Part model, mm, in its own coordinate system. A direction names the side the tool comes from. Coordinates: 2 decimals unless noted, no trailing zeros. Order: outer loops, then holes, each group sorted by start corner. A loop starts at its lowest first (then second) coordinate and runs counter-clockwise, first axis right, second up. Notation, with made-up numbers: (-6, 10.5) - (2, 10.5) arc R20 cw to (2, 42.5) - close; hole circle Ø9 at (-40, 30). An arc over 180 degrees is marked (long way). Use a Markdown table: item, result. Add a question column.
1) Saw through at B-B on x = 3. List the corners of the cut face in (y, z).
2) Drop flat-ended pins along their axis: P1, Ø6, axis at x = -5, y = 3, coming from the +Z side; P2, Ø2, axis at x = -3, y = -4, coming from the -Z side. Give the stop position or say it passes through.
3) Wall check: L1, parallel to Y at x = 1.5, z = 1.8; L2, parallel to Y at x = 1.75, z = 0.5; L3, parallel to X at y = 4.5, z = 0.7. Give the ranges that are in metal, low to high. Write a range as [from, to].
4) Tool access for faces 1 (the face through (1.39, 1.52, 2)), 2 (the face through (3.138, -3.702, 1.268)), 3 (the face through (-3.88, -7.31, 2)), 4 (the face through (-4.53, -7.12, 1.27)): list every direction of +Z, -Z, +X, -X, +Y, -Y with a clear straight run to the whole face (end or side of a thin tool).
5) Saw through at D-D on z = 2.15. List the corners of the cut face in (x, y), then the cut area to 3 significant figures.
6) Saw through at A-A on z = 0.3. List the corners of the cut face in (x, y), then the cut area to 3 significant figures.
7) Saw through at C-C on y = -6. List the corners of the cut face in (x, z), then the cut area to 3 significant figures.
```python
from build123d import *

# Parameters (mm, degrees)
F1_DEPTH = 2.54
F2_SIZE  = 1.0922
F3_SIZE  = 1.0922


with BuildPart() as f1:
    # F0 (on Top) → F1 (new body)
    with BuildSketch(Plane.XY):
        Polygon((3.7357374094, 2.0727487281), (1.6156566562, 6.3129104674), (-0.688809203, 5.7773781009), (0, 3.146545263), (-3.5388784017, 1.3378473232), (-1.3465175871, -4.636336118), (-7.8139826655, -9.6787661314), (-5.0735310651, -18.2837825269), (5.5594188161, -7.8152595088), (0.6475421183, 0.5286511673), align=None)
    extrude(amount=F1_DEPTH)

    # F2
    f2_edges = [f1.edges().sort_by_distance(p)[0] for p in [
        (3.10348, -3.643304, 2.54),
        (2.19164, 1.3007, 2.54),
        (2.675697, 4.19283, 2.54),
        (0.463424, 6.045144, 2.54),
        (-0.344405, 4.461962, 2.54),
        (-1.769439, 2.242196, 2.54),
        (-2.442698, -1.649244, 2.54),
        (-4.58025, -7.157551, 2.54),
        (-6.443757, -13.981274, 2.54),
        (0.242944, -13.049521, 2.54),
    ]]
    chamfer(f2_edges, length=F2_SIZE)

    # F3
    f3_edges = [f1.edges().sort_by_distance(p)[0] for p in [
        (3.10348, -3.643304, 0),
        (2.19164, 1.3007, 0),
        (2.675697, 4.19283, 0),
        (0.463424, 6.045144, 0),
        (-0.344405, 4.461962, 0),
        (-1.769439, 2.242196, 0),
        (-2.442698, -1.649244, 0),
        (-4.58025, -7.157551, 0),
        (-6.443757, -13.981274, 0),
        (0.242944, -13.049521, 0),
    ]]
    chamfer(f3_edges, length=F3_SIZE)


solid = f1.part
```
Results are:
| question | item | result |
|---|---|---|
| 1 | outline | (-10.34, 1.09) - (-8.8, 0) - (-5.62, 0) - (-3.47, 1.09) - (-3.47, 1.45) - (-5.62, 2.54) - (-8.8, 2.54) - (-10.34, 1.45) - close; (1.7, 1.09) - (2.32, 0.54) - (3.54, 1.09) - (3.54, 1.45) - (2.32, 2) - (1.7, 1.45) - close |
| 2 | P1 | z = 2.09 |
| 2 | P2 | through |
| 3 | L1 | [-11.32, -1.61], [1.35, 5.76] |
| 3 | L2 | [-10.73, -2.51], [1.74, 4.72] |
| 3 | L3 | [0.05, 2.08] |
| 4 | face 1 | +Z, +X |
| 4 | face 2 | +Z, -Z, +X |
| 4 | face 3 | +Z, -X |
| 4 | face 4 | +Z, -Z, -X |
| 5 | outline | (-7, -9.93) - (-4.75, -16.98) - (4.68, -7.7) - (-0.34, 0.82) - (2.79, 2.39) - (1.24, 5.5) - (0.17, 5.26) - (0.82, 2.78) - (-2.67, 1) - (-0.51, -4.88) - close |
| 5 | area | 96.3 mm2 |
| 6 | outline | (-6.89, -9.96) - (-4.71, -16.81) - (4.56, -7.68) - (-0.47, 0.86) - (2.67, 2.43) - (1.19, 5.4) - (0.28, 5.19) - (0.93, 2.73) - (-2.55, 0.95) - (-0.4, -4.91) - close |
| 6 | area | 91.0 mm2 |
| 7 | outline | (-3.1, 1.09) - (-1.32, 0) - (3.22, 0) - (4.49, 1.09) - (4.49, 1.45) - (3.22, 2.54) - (-1.32, 2.54) - (-3.1, 1.45) - close |
| 7 | area | 15.9 mm2 |
